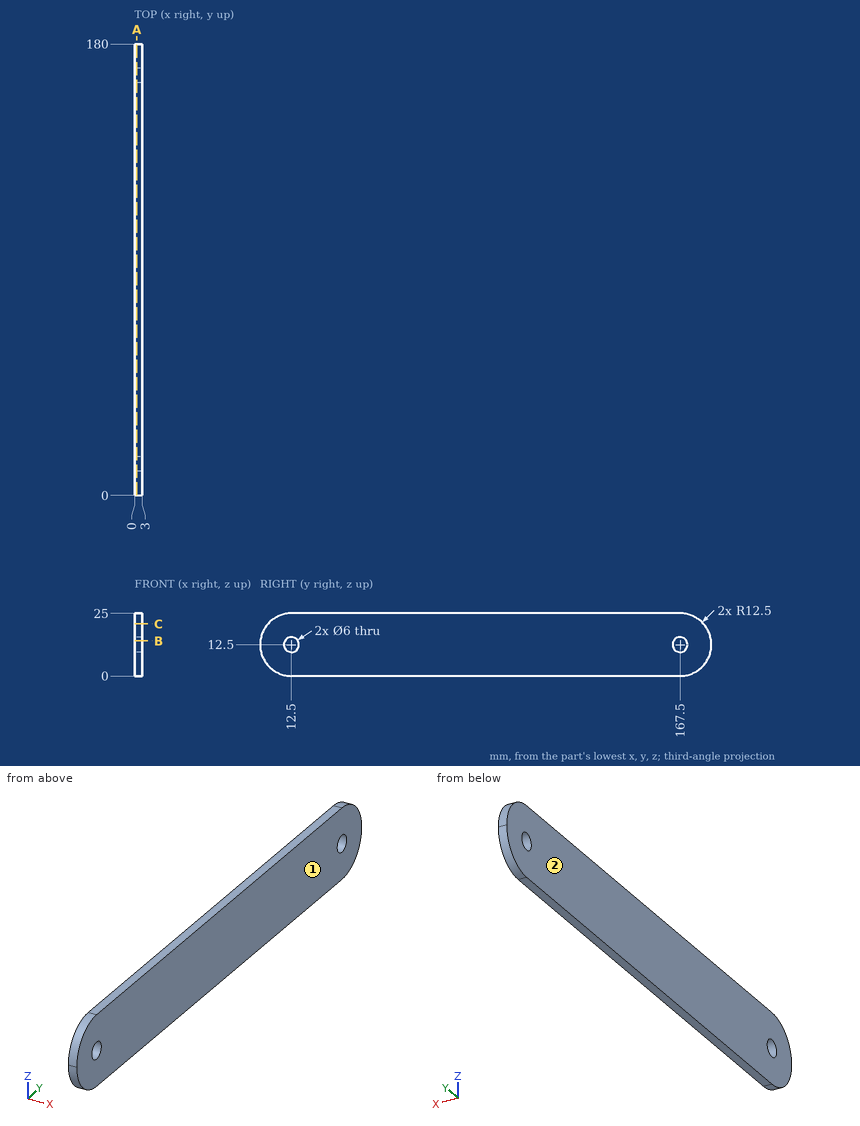
The drawing under review shows one solid part. Ordinate dimensions are in mm from its lowest x, y, z. Give positions to 0.01 mm unless a question says otherwise; leave off trailing zeros. Loops run counter-clockwise (first coordinate to the right, second up) from the corner with the lowest first, then second, coordinate; pieces in that order, holes last. Notation, with made-up numbers: M 35.25,49.25 L 78.25,49.25 A33 ccw 78.25,83.25 Z; hole C 60.5,45.5 d6. An arc over 180 degrees is marked long. One line per item, written item: value. Start each with the question number.
Q1. For L1, parallel to Z at x = 1.6, y = 167.5; L2, parallel to Y at x = 1.6, z = 10.25; L3, parallel to Z at x = 1.9, y = 165, list the stretches that pass through material, from the lowest coordinate up.
Q2. Draft analysis for pull direction X (two halves, no side actions). For the marked faces 1 and 2, state which applies: released by +X, released by -X, zero draft, split by the parting line, or undercut.
Q3. Add section A-A (x = 0.9). Give the boundary of the cut face in (y, z).
Q4. Add section B-B (z = 14). Give the boundary of the cut face in (x, y), and give its area (3 significant figures).
Q5. Add section C-C (z = 20.75). Give the boundary of the cut face in (x, y), and give its area (3 significant figures).
Reply:
1. L1: 0 to 9.5, 15.5 to 25
1. L2: 0.2 to 10.52, 14.48 to 165.52, 169.48 to 179.8
1. L3: 0 to 10.84, 14.16 to 25
2. face 1: released by +X
2. face 2: released by -X
3. outline: M 0,12.5 A12.5 ccw 12.5,0 L 167.5,0 A12.5 ccw 180,12.5 A12.5 ccw 167.5,25 L 12.5,25 A12.5 ccw Z; hole C 12.5,12.5 d6; hole C 167.5,12.5 d6
4. outline: M 0,0.09 L 3,0.09 L 3,9.9 L 0,9.9 Z; M 0,15.1 L 3,15.1 L 3,164.9 L 0,164.9 Z; M 0,170.1 L 3,170.1 L 3,179.91 L 0,179.91 Z
4. area: 508 mm²
5. outline: M 0,3.11 L 3,3.11 L 3,176.89 L 0,176.89 Z
5. area: 521 mm²
